Geometry check sheet. Reference: the model listing, model coordinates, mm. Face numbers are marked on the shaded views. Coordinates: 2 decimals unless noted, no trailing zeros. Write each loop counter-clockwise with the first axis right and the second up, starting at its lowest first coordinate (ties: lowest second). Pieces come first, ordered by that corner, then holes. Notation, with made-up numbers: (75.5, 9.25) -> (98.5, 9.25) arc R19 ccw to (98.5, 36.25) -> close; hole circle Ø10 at (-23.5, 0). An arc over 180 degrees is marked (long way). Answer as CSV lines item,"result".
```python
from build123d import *

# Parameters (mm, degrees)
ESQUISSE1_R          = 17.25
ESQUISSE1_R_2        = 15
BASE_EXTRUSION_DEPTH = 22
CONG_1_R             = 0.5
CHANFREIN1_SIZE      = 1


with BuildPart() as part:
    # Esquisse1 → Base-Extrusion (new body)
    with BuildSketch(Plane.XY):
        Circle(ESQUISSE1_R)
        Circle(ESQUISSE1_R_2, mode=Mode.SUBTRACT)
    extrude(amount=BASE_EXTRUSION_DEPTH)

    # Congé1
    cong_1_edges = [part.edges().sort_by_distance(p)[0] for p in [
        (-17.25, 0, 0),
        (-17.25, 0, 22),
    ]]
    fillet(cong_1_edges, radius=CONG_1_R)

    # Chanfrein1
    chanfrein1_edges = [part.edges().sort_by_distance(p)[0] for p in [
        (-15, 0, 0),
        (-15, 0, 22),
    ]]
    chamfer(chanfrein1_edges, length=CHANFREIN1_SIZE)


solid = part.part
```
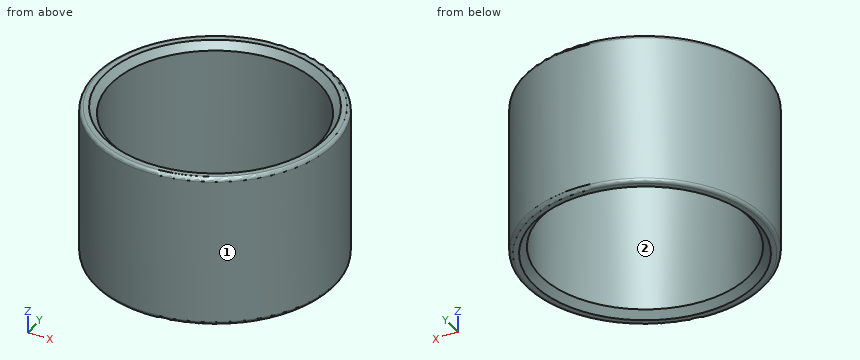
Item 1: Depth check by flat-ended pin: pin 1 Ø8 at (x, z) = (-5, 3) entering from -Y; pin 2 Ø12 at (x, z) = (8.5, 9.5) entering from +Y; pin 3 Ø4 at (y, z) = (-9.5, 6.5) entering from +X. Enter the tip coordinate at first touch or a pass-through.
Responses:
pin 1,"stops at y = -17.22"
pin 2,"stops at y = 17.07"
pin 3,"stops at x = 15.53"
Item 2: Cross-section at C-C, the plane z = 2.5. Record the cut outline in (x, y), plus the area to 3 significant figures.
Responses:
outline,"circle Ø34.5 at (0, 0); hole circle Ø30 at (0, 0)"
area,"228 mm2"
Item 3: Release check for a two-part mould opening along X. For the marked faces 1 and 2 record: +X half, -X half, draft (parallel to the pull), parting line (faces both ways), or undercut.
Responses:
face 1,"parting line"
face 2,"undercut"
Item 4: Thickness scan on probe 1 along Y at (x, z) = (0, 12.5); probe 2 along X at (y, z) = (13.5, 16.25); probe 3 along X at (y, z) = (13, 17). Record the ranges inside material, lowest first.
Responses:
probe 1,"y = -17.25 to -15, 15 to 17.25"
probe 2,"x = -10.74 to -6.54, 6.54 to 10.74"
probe 3,"x = -11.34 to -7.48, 7.48 to 11.34"
Item 5: Cross-section at A-A, the plane y = 0. Record the cut outline in (x, z), plus the area to 3 significant figures.
Responses:
outline,"(-17.25, 0.5) arc R0.5 ccw to (-16.75, 0) -> (-16, 0) -> (-15, 1) -> (-15, 21) -> (-16, 22) -> (-16.75, 22) arc R0.5 ccw to (-17.25, 21.5) -> close; (15, 1) -> (16, 0) -> (16.75, 0) arc R0.5 ccw to (17.25, 0.5) -> (17.25, 21.5) arc R0.5 ccw to (16.75, 22) -> (16, 22) -> (15, 21) -> close"
area,"96.8 mm2"
